CAD build for the part. Positions are in the model's coordinates, mm. A direction names the side the tool comes from. Coordinates: 2 decimals unless noted, no trailing zeros. Order: outer loops, then holes, each group sorted by start corner. A loop starts at its lowest first (then second) coordinate and runs counter-clockwise, first axis right, second up. Notation, with made-up numbers: (16.5, 73.5) - (51.5, 73.5) arc R21 ccw to (51.5, 108.5) - close; hole circle Ø4 at (-0.75, 7.25). An arc over 180 degrees is marked (long way). Return JSON: item names as keys, results as strings.
from build123d import *

# Parameters (mm, degrees)
CUT_EXTRUDE_START   = -15
CUT_EXTRUDE_1_DEPTH = 15


with BuildPart() as part:
    # 草图1 → 旋转1 (revolve)
    with BuildSketch(Plane(origin=(0, 0, 0), x_dir=(1, 0, 0), z_dir=(0, 1, 0)), mode=Mode.PRIVATE) as revolve_1_sk:
        Polygon((-85, 10), (-85, 47.75), (-75, 47.75), (-75, 41.078952229), (75, 41.078952229), (75, 47.75), (85, 47.75), (85, 10), align=None)
    revolve(revolve_1_sk.sketch.rotate(Axis((-58.327347129, 0, 0), (1, 0, 0)), 180), axis=Axis((-58.327347129, 0, 0), (1, 0, 0)))

    # 草图2 → 切除-拉伸1 (cut)
    with BuildSketch(Plane(origin=(85, 0, 0), x_dir=(0, 0, -1), z_dir=(1, 0, 0)).offset(CUT_EXTRUDE_START)):
        with BuildLine():
            Line((9.797958971, 2), (13.797958971, 2))
            Line((13.797958971, 2), (13.797958971, -2))
            Line((13.797958971, -2), (9.797958971, -2))
            ThreePointArc((9.797958971, -2), (10, 0), (9.797958971, 2))
        make_face()
    extrude(amount=CUT_EXTRUDE_1_DEPTH, mode=Mode.SUBTRACT)


solid = part.part
Item 1: Which spindle directions (+Z, -Z, +X, -X, +Y, -Y) get a long thin tool onto all of the face, cutting with end or side? Do faces 4 (the cylindrical face through (-79.93, 42.362, 22.034)), 5 (the flat face through (77, -2, -12)), 6 (the flat face through (75, -36, -21)). Say none if no direction does.
Findings below:
{"face 4": "+X, -X", "face 5": "+X", "face 6": "none"}
Item 2: Band-saw the part on D-D, the plane x = -55. List the corners of the cut face in (y, z).
Findings below:
{"outline": "circle Ø82.16 at (0, 0); hole circle Ø20 at (0, 0)"}
Item 3: Drop flat-ended pins along their axis: P1, Ø6, axis at x = 49.5, y = 24.5, coming from the -Z side; P2, Ø1, axis at x = 14.5, y = -21.5, coming from the -Z side; P3, Ø12, axis at x = -48, y = -34.5, coming from the -Z side. Give the stop position or say it passes through.
Findings below:
{"P1": "stops at z = -35", "P2": "stops at z = -35.31", "P3": "stops at z = -29.58"}
Item 4: Wall check: L1, parallel to X at y = 20.5, z = -39; L2, parallel to Y at x = 37, z = 0; L3, parallel to Z at x = -73.5, y = 7.5. Give the ranges that are in metal, low to high. Write a range as [from, to].
Findings below:
{"L1": "x = [-85, -75], [75, 85]", "L2": "y = [-41.08, -10], [10, 41.08]", "L3": "z = [-40.39, -6.61], [6.61, 40.39]"}
Item 5: Band-saw the part on C-C, the plane y = 22. List the corners of the cut face in (x, z), then the cut area to 3 significant figures.
Findings below:
{"outline": "(-85, -42.38) - (-75, -42.38) - (-75, -34.69) - (75, -34.69) - (75, -42.38) - (85, -42.38) - (85, 42.38) - (75, 42.38) - (75, 34.69) - (-75, 34.69) - (-75, 42.38) - (-85, 42.38) - close", "area": "12,100 mm²"}
Item 6: Mould opens along X. For faces 1 (the flat face through (-85, -11, 1)), 2 (the flat face through (77, 0, -13.798)), 3 (the cylindrical face through (1.05, 40.1, -8.91)) say: released by +X, released by -X, zero draft, split by the parting line, or undercut.
Findings below:
{"face 1": "released by -X", "face 2": "zero draft", "face 3": "undercut"}
Item 7: Band-saw the part on B-B, the plane y = 0. List the corners of the cut face in (x, z).
Findings below:
{"outline": "(-85, -47.75) - (-75, -47.75) - (-75, -41.08) - (75, -41.08) - (75, -47.75) - (85, -47.75) - (85, -13.8) - (70, -13.8) - (70, -10) - (-85, -10) - close; (-85, 10) - (85, 10) - (85, 47.75) - (75, 47.75) - (75, 41.08) - (-75, 41.08) - (-75, 47.75) - (-85, 47.75) - close"}
Item 8: Band-saw the part on A-A, the plane z = 0. List the corners of the cut face in (x, y).
Findings below:
{"outline": "(-85, -47.75) - (-75, -47.75) - (-75, -41.08) - (75, -41.08) - (75, -47.75) - (85, -47.75) - (85, -10) - (-85, -10) - close; (-85, 10) - (85, 10) - (85, 47.75) - (75, 47.75) - (75, 41.08) - (-75, 41.08) - (-75, 47.75) - (-85, 47.75) - close"}
